```python
from build123d import *

# Parameters (mm, degrees)
BOSS_EXTRUDE1_DEPTH = 1.524


with BuildPart() as part:
    # Sketch1 → Boss-Extrude1 (new body)
    with BuildSketch(Plane.XY):
        with BuildLine():
            Line((0, 30.238088669), (-1.524, 30.238088669))
            Line((-1.524, 30.238088669), (-1.524, 30.790634065))
            ThreePointArc((-1.524, 30.790634065), (-4.57902006, 29.852179907), (-3.574419861, 26.818267876))
            ThreePointArc((-3.574419861, 26.818267876), (22.721404873, 15.60835362), (45.010506388, -2.289370529))
            ThreePointArc((45.010506388, -2.289370529), (46.184159064, -2.824291441), (47.467988652, -2.700264938))
            ThreePointArc((47.467988652, -2.700264938), (46.368179039, -2.362168668), (45.427846615, -1.69909612))
            ThreePointArc((45.427846615, -1.69909612), (25.999332487, 14.287912382), (4.180950484, 26.818267876))
            ThreePointArc((4.180950484, 26.818267876), (3.159648615, 26.95869619), (2.318491113, 27.55470934))
            ThreePointArc((2.318491113, 27.55470934), (1.568114485, 29.962053436), (0, 31.936740157))
            Line((0, 31.936740157), (0, 30.238088669))
        make_face()
    extrude(amount=BOSS_EXTRUDE1_DEPTH)


solid = part.part
```
Verification items for the finished model (mm, model axes). A direction names the side the tool comes from. Give positions to 0.01 mm unless a question says otherwise; leave off trailing zeros. Loops run counter-clockwise (first coordinate to the right, second up) from the corner with the lowest first, then second, coordinate; pieces in that order, holes last.
1. Section check B-B, the plane x = 1. Enter the section's corners in (y, z), then the cut area to 3 significant figures.
2. Mould release check, pull along X, two halves, no side actions. Record for faces 1 (the cylindrical face through (26.289, 14.087, 0.751)), 2 (the flat face through (0, 31, 1)), 3 (the flat face through (13, 21, 1.524)), 4 (the cylindrical face through (22.4, 15.8, 0.8)): released by +X, released by -X, zero draft, split by the parting line, or undercut.
3. Set-up check for faces 5 (the cylindrical face through (46.17, -2.82, 0.75)), 6 (the flat face through (-1, 30.238, 1)): record each of +Z, -Z, +X, -X, +Y, -Y from which the full face is reachable in a straight line by a thin tool's end or side.
4. Thickness scan on line 1 (X direction, y = 30.5, z = 1.15); line 2 (X direction, y = 27.5, z = 0.45); line 3 (Y direction, x = 19, z = 0.25). Record the ranges inside material, lowest first.
5. Section check C-C, the plane y = 5. Enter the section's corners in (x, z), then the cut area to 3 significant figures.
6. Section check A-A, the plane z = 0.7. Enter the section's corners in (x, y), then the cut area to 3 significant figures.
Geometry says:
1. outline: (25.46, 0) - (30.86, 0) - (30.86, 1.52) - (25.46, 1.52) - close
1. area: 8.23 mm2
2. face 1: released by +X
2. face 2: undercut
2. face 3: zero draft
2. face 4: released by -X
3. face 5: +Z, -Z, -Y
3. face 6: +Z, -Z, +Y
4. line 1: x = -4.08 to -1.52, 0 to 1.25
4. line 2: x = -4.39 to 2.37
4. line 3: y = 17.74 to 18.85
5. outline: (37.39, 0) - (38.08, 0) - (38.08, 1.52) - (37.39, 1.52) - close
5. area: 1.05 mm2
6. outline: (-3.57, 26.82) arc R104.81 cw to (45.01, -2.29) arc R2.49 ccw to (47.47, -2.7) arc R3.66 cw to (45.43, -1.7) arc R150.64 ccw to (4.18, 26.82) arc R2.17 cw to (2.32, 27.55) arc R6.87 ccw to (0, 31.94) - (0, 30.24) - (-1.52, 30.24) - (-1.52, 30.79) arc R2.24 ccw (long way) to start
6. area: 80.7 mm2
